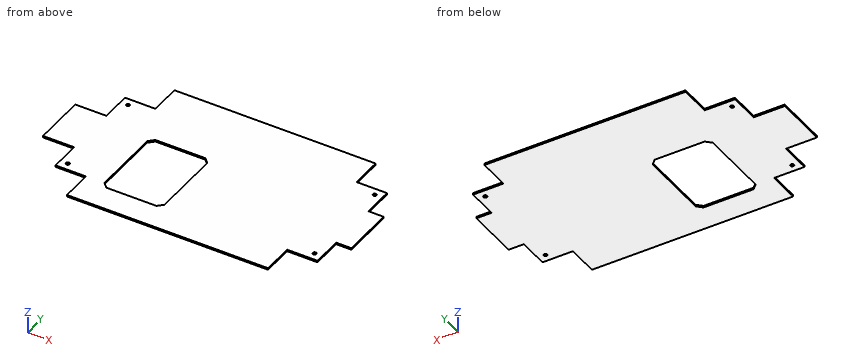
```python
from build123d import *

# Parameters (mm, degrees)
BOSS_EXTRU_1_DEPTH      = 3.3
ESQUISSE2_W             = 401.8
ESQUISSE2_H             = 6.35
ENL_V_MAT_EXTRU_1_DEPTH = 643.284432709
D_GAGEMENT_1_41_D       = 7.14248
ESQUISSE5_W             = 401.8
ESQUISSE5_H             = 1.35
BOSS_EXTRU_2_DEPTH      = 3.3
ESQUISSE6_W             = 120
ESQUISSE6_H             = 160
ENL_V_MAT_EXTRU_2_DEPTH = 641.514024046
CHANFREIN1_SIZE         = 10


with BuildPart() as part:
    # Esquisse1 → Boss.-Extru.1 (new body)
    with BuildSketch(Plane.XY):
        Polygon((-615.95, 52.7), (-615.95, -52.7), (-553.8, -52.7), (-553.8, -113.5), (-493, -113.5), (-493, -174.3), (-91.2, -174.3), (-91.2, -113.5), (-30.4, -113.5), (-30.4, -52.7), (0, -52.7), (0, 52.7), (-30.4, 52.7), (-30.4, 113.5), (-91.2, 113.5), (-91.2, 182), (-493, 182), (-493, 113.5), (-553.8, 113.5), (-553.8, 52.7), align=None)
    extrude(amount=BOSS_EXTRU_1_DEPTH)

    # Esquisse2 → Enlèv. mat.-Extru.1 (cut, through all)
    with BuildSketch(Plane.XY.offset(3.3)):
        with Locations((-292.1, 178.825)):
            Rectangle(ESQUISSE2_W, ESQUISSE2_H)
    extrude(amount=-ENL_V_MAT_EXTRU_1_DEPTH, mode=Mode.SUBTRACT)

    # Dégagement 1/41 (through all)
    with Locations(Plane(origin=(0, 0, 0), x_dir=(-1, 0, 0), z_dir=(0, 0, -1))):
        with Locations((45.6, 98.3), (45.6, -98.3), (538.6, -98.3), (538.6, 98.3)):
            Hole(D_GAGEMENT_1_41_D / 2)

    # Esquisse5 → Boss.-Extru.2 (add, through all)
    with BuildSketch(Plane.XY.offset(3.3)):
        with Locations((-292.1, -174.975)):
            Rectangle(ESQUISSE5_W, ESQUISSE5_H)
    extrude(amount=-BOSS_EXTRU_2_DEPTH)

    # Esquisse6 → Enlèv. mat.-Extru.2 (cut, through all)
    with BuildSketch(Plane(origin=(0, 0, 0), x_dir=(-1, 0, 0), z_dir=(0, 0, -1))):
        with Locations((396.566519887, -42.768394731)):
            Rectangle(ESQUISSE6_W, ESQUISSE6_H)
    extrude(amount=-ENL_V_MAT_EXTRU_2_DEPTH, mode=Mode.SUBTRACT)

    # Chanfrein1
    chanfrein1_edges = [part.edges().sort_by_distance(p)[0] for p in [
        (-336.566519887, -122.768394731, 1.65),
        (-336.566519887, 37.231605269, 1.65),
        (-456.566519887, 37.231605269, 1.65),
        (-456.566519887, -122.768394731, 1.65),
    ]]
    chamfer(chanfrein1_edges, length=CHANFREIN1_SIZE)


solid = part.part
```
Here's how the part is built. I have some questions about the finished solid (model axes, mm). Coordinates: 2 decimals unless noted, no trailing zeros. Order: outer loops, then holes, each group sorted by start corner. A loop starts at its lowest first (then second) coordinate and runs counter-clockwise, first axis right, second up.
1) Imagine slicing it at B-B on x = -74. List the corners of the cut face in (y, z) for me.
2) Will these pins go through, and if not, where does the flat tip stop? pin 1 (1.6 mm diameter, centred on x = -21.5, z = 2, fed in from -Y); pin 2 (1 mm diameter, centred on y = 132, z = 1.5, fed in from +X); pin 3 (8 mm diameter, centred on x = -45.6, y = 98.3, fed in from -Z); pin 4 (1.5 mm diameter, centred on y = 84, z = 2.5, fed in from -X).
3) Imagine slicing it at C-C on y = -130.5. List the corners of the cut face in (x, z) for me, and give its area (3 significant figures).
4) Imagine slicing it at A-A on z = 2.4. State how many separate pieces and enclosed holes the cut face has, and give its area (3 significant figures).
5) I need wall thicknesses on line 1 (Y direction, x = -45.6, z = 2.05); line 2 (X direction, y = -2, z = 1.85); line 3 (X direction, y = 147.5, z = 2.95). Which ranges of each line are inside material? Lowest first, please.
Response values:
1. outline: (-113.5, 0) - (113.5, 0) - (113.5, 3.3) - (-113.5, 3.3) - close
2. pin 1: stops at y = -52.7
2. pin 2: stops at x = -91.2
2. pin 3: stops at z = 0
2. pin 4: stops at x = -553.8
3. outline: (-493, 0) - (-91.2, 0) - (-91.2, 3.3) - (-493, 3.3) - close
3. area: 1,330 mm2
4. separate pieces: 1
4. enclosed holes: 5
4. area: 159,000 mm2
5. line 1: y = -113.5 to -101.87, -94.73 to 94.73, 101.87 to 113.5
5. line 2: x = -615.95 to -456.57, -336.57 to 0
5. line 3: x = -493 to -91.2
